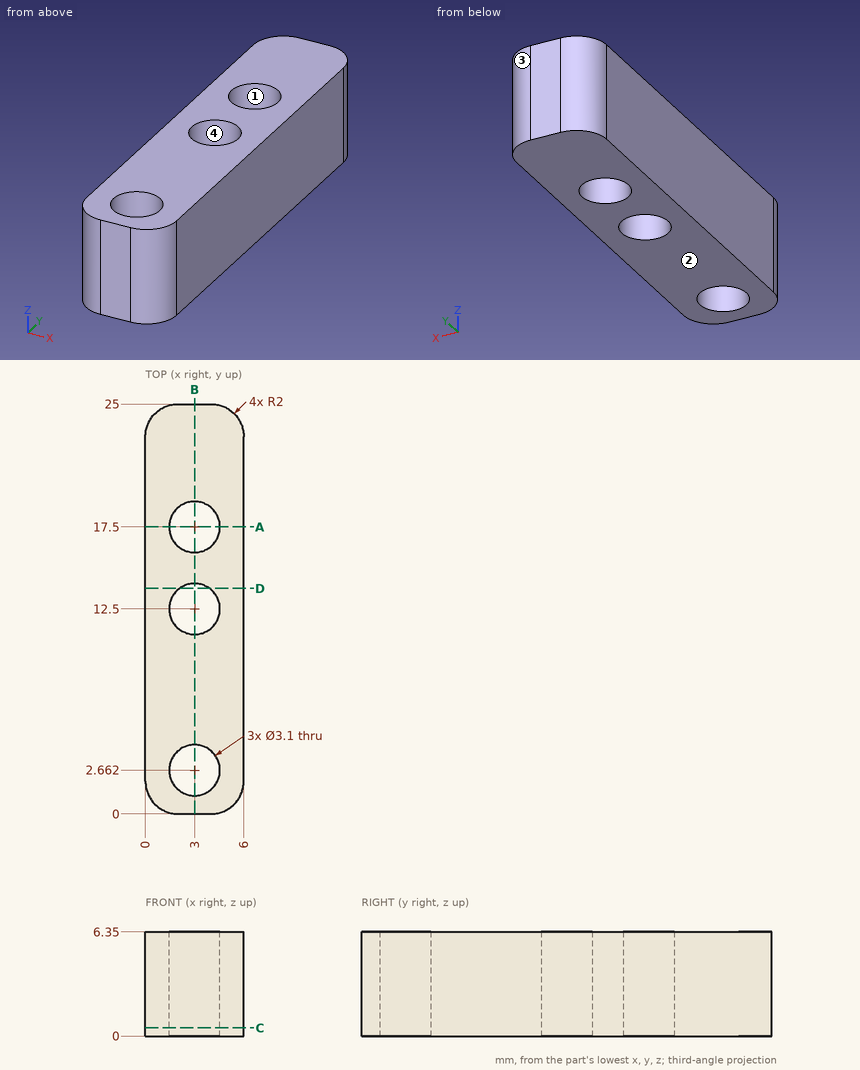
Input: dimensioned drawing with shaded views. Units: mm. Origin: part minimum x, y, z. Coordinates: 2 decimals unless noted, no trailing zeros. Loops run counter-clockwise (first coordinate to the right, second up) from the corner with the lowest first, then second, coordinate; pieces in that order, holes last. Notation, with made-up numbers: M 47,9 L 68,9 A27 cw 68,29 Z; hole C -18,89.5 d5. An arc over 180 degrees is marked long. One line per item, written item: value. Start each with the question number.
1) Cut plane C-C (z = 0.5). Return loops of the section in (x, y), then the cut area to 3 significant figures.
2) Cut plane A-A (y = 17.5). Return loops of the section in (x, z).
3) Cut plane B-B (x = 3). Return loops of the section in (y, z).
4) Draft query along Y for the marked faces 1, 2, 3 and 4. Return one class per face: released by +Y, released by -Y, zero draft, split by the parting line, or undercut.
5) Cut plane D-D (y = 13.75). Return loops of the section in (x, z).
6) Material intervals for L1, parallel to Y at x = 3, z = 2; L2, parallel to Y at x = 2.5, z = 5.5 (1 decimal); L3, parallel to X at y = 16.5, z = 4.5 (1 decimal), sorted ascending. Write a range as from..to.
Evaluation:
1. outline: M 0,2 A2 ccw 2,0 L 4,0 A2 ccw 6,2 L 6,23 A2 ccw 4,25 L 2,25 A2 ccw 0,23 Z; hole C 3,2.66 d3.1; hole C 3,12.5 d3.1; hole C 3,17.5 d3.1
1. area: 124 mm^2
2. outline: M 0,0 L 1.45,0 L 1.45,6.35 L 0,6.35 Z; M 4.55,0 L 6,0 L 6,6.35 L 4.55,6.35 Z
3. outline: M 0,0 L 1.11,0 L 1.11,6.35 L 0,6.35 Z; M 4.21,0 L 10.95,0 L 10.95,6.35 L 4.21,6.35 Z; M 14.05,0 L 15.95,0 L 15.95,6.35 L 14.05,6.35 Z; M 19.05,0 L 25,0 L 25,6.35 L 19.05,6.35 Z
4. face 1: undercut
4. face 2: zero draft
4. face 3: released by +Y
4. face 4: undercut
5. outline: M 0,0 L 2.08,0 L 2.08,6.35 L 0,6.35 Z; M 3.92,0 L 6,0 L 6,6.35 L 3.92,6.35 Z
6. L1: 0..1.11, 4.21..10.95, 14.05..15.95, 19.05..25
6. L2: 0..1.2, 4.1..11, 14..16, 19..25
6. L3: 0..1.8, 4.2..6
